CAD build for the part. Positions are in the model's coordinates, mm. A direction names the side the tool comes from. Round coordinates to 2 decimals unless told otherwise and drop trailing zeros. Write each loop counter-clockwise with the first axis right and the second up, starting at its lowest first coordinate (ties: lowest second). Pieces come first, ordered by that corner, then holes. Notation, with made-up numbers: (40, 20.25) - (58, 20.25) arc R11 ccw to (58, 29.25) - close; hole circle Ø5 at (39, 6). An arc over 180 degrees is marked (long way). Use one line per item in the form item = value. Start each with the question number.
Item 1: Band-saw the part on C-C, the plane x = 19.05. List the corners of the cut face in (y, z), and give its area (3 significant figures).
Item 2: Band-saw the part on B-B, the plane z = 0. List the corners of the cut face in (x, y), and give its area (3 significant figures).
Item 3: Pull direction X, two halves, no side cores. Call faces 1 (the cylindrical face through (-23.046, 6.465, 0.176)), 2 (the flat face through (0, 9, 15)), 3 (the flat face through (-24, 2, 0)): +X half, -X half, draft (parallel to the pull), parting line (faces both ways), or undercut.
Item 4: Drill centre lines: L1, parallel to X at y = 2.25, z = 0; L2, parallel to Z at x = 19.05, y = 5.25; L3, parallel to Z at x = -12.5, y = 2.4. Where is each one in solid material? Low to high.
Item 5: Pin check, flat tips, straight feed: pin 1 (4.5 mm diameter, centred on x = 12.5, z = 4, fed in from -Y); pin 2 (2.5 mm diameter, centred on y = 5.5, z = -16, fed in from -X); pin 3 (2.5 mm diameter, centred on y = 7.5, z = 15, fed in from +X). Stop position of each tip, or through.
Item 6: Tool access for faces 4 (the cylindrical face through (10.502, 2.246, 5.088)), 5 (the flat face through (-2.5, 6, 15)), 6 (the flat face through (0, 6, -12.5)), 7 (the flat face through (2.5, 6, 15)), 8 (the cylindrical face through (15.876, 6.465, -2.434)): list every direction of +Z, -Z, +X, -X, +Y, -Y with a clear straight run to the whole face (end or side of a thin tool).
Item 7: Band-saw the part on D-D, the plane z = -5. List the corners of the cut face in (x, y).
Item 8: Band-saw the part on A-A, the plane y = 3.25. List the corners of the cut face in (x, z), and give its area (3 significant figures).
Autodesk Inventor part; units mm, degrees
ref_plane "YZ Plane" through (0, 0, 0) normal (1, 0, 0) x (0, 1, 0)
ref_plane "XZ Plane" through (0, 0, 0) normal (0, 1, 0) x (-1, 0, 0)
ref_plane "XY Plane" through (0, 0, 0) normal (0, 0, 1) x (1, 0, 0)
sketch "Sketch1" plane through (0, 0, 0) normal (0, 1, 0) x (-1, 0, 0)
  line L0 (-24, 17.5) -> (24, 17.5)
  line L1 (24, 17.5) -> (24, -17.5)
  line L2 (24, -17.5) -> (-24, -17.5)
  line L3 (-24, -17.5) -> (-24, 17.5)
  line L4 (-24, 17.5) -> (24, -17.5) construction
  line L5 (24, 17.5) -> (-24, -17.5) construction
  point P0 (0, 0)
  dimension "d0" = 48
  dimension "d1" = 35
extrude "Extrusion1" add sketch "Sketch1" along normal blind 4
sketch "Sketch2" plane through (0, 4, 0) normal (0, 1, 0) x (1, 0, 0)
  line L0 (0, 0) -> (-5.2635, 0) construction
  line L1 (-5.2635, 0) -> (-5.2635, 9.5172) construction
  line L2 (-5.2635, 9.5172) -> (0, 9.5172) construction
  line L3 (0, 9.5172) -> (0, 0) construction
  circle A0 centre (-19.05, 0) radius 1
  circle A1 centre (19.05, 0) radius 1
  circle A2 centre (-19.05, 0) radius 4
  circle A3 centre (19.05, 0) radius 4
  line L4 (-24, -17.5) -> (24, -17.5)
  line L5 (0, -17.5) -> (-2.5, -17.5)
  line L6 (-2.5, -17.5) -> (-2.5, -12.5)
  line L7 (-2.5, -12.5) -> (0, -12.5)
  line L8 (0, -12.5) -> (0, -17.5)
  line L9 (2.5, -17.5) -> (2.5, -12.5)
  line L10 (2.5, -12.5) -> (0, -12.5)
  line L11 (-2.5, 17.5) -> (-2.5, 12.5)
  line L12 (-2.5, 12.5) -> (0, 12.5)
  line L13 (2.5, 17.5) -> (2.5, 12.5)
  line L14 (2.5, 12.5) -> (0, 12.5)
  line L15 (24, 17.5) -> (-24, 17.5)
  dimension "d4" = 2
  dimension "d5" = 19.05
  dimension "d6" = 3
  dimension "d7" = 3
  dimension "d8" = 2.5
  dimension "d9" = 5
extrude "Extrusion2" add sketch "Sketch2" along normal blind 5
chamfer "Chamfer1" distance 15 angle 45 4 edges at (24, 2, -17.5) (24, 2, 17.5) (-24, 2, 17.5) (-24, 2, -17.5)
sketch "Sketch4" plane through (19.05, 9, 0) normal (0, 1, 0) x (1, 0, 0)
  circle A0 centre (0, 0) radius 1
  circle A1 centre (-38.1, 0) radius 1
  point P0 (-19.05, 0)
extrude "Extrusion3" cut sketch "Sketch4" against normal through all
sketch "Sketch7" plane through (0, 0, 0) normal (0, -1, 0) x (1, 0, 0)
  line L0 (14.5, -3) -> (10.5, -3)
  line L1 (10.5, -3) -> (10.5, -7)
  line L2 (10.5, -7) -> (14.5, -7)
  line L3 (14.5, -7) -> (14.5, -3)
  line L4 (0, -6.5734) -> (0, 0) construction
  line L5 (0, 0) -> (6.1677, 0) construction
  line L6 (-14.5, -3) -> (-10.5, -3)
  line L7 (-10.5, -3) -> (-10.5, -7)
  line L8 (-10.5, -7) -> (-14.5, -7)
  line L9 (-14.5, -7) -> (-14.5, -3)
  line L10 (14.5, 3) -> (10.5, 3)
  line L11 (10.5, 3) -> (10.5, 7)
  line L12 (10.5, 7) -> (14.5, 7)
  line L13 (14.5, 7) -> (14.5, 3)
  line L14 (-10.5, 7) -> (-14.5, 7)
  line L15 (-10.5, 3) -> (-10.5, 7)
  line L16 (-14.5, 3) -> (-10.5, 3)
  line L17 (-14.5, 7) -> (-14.5, 3)
  circle A0 centre (12.5, -5) radius 2
  circle A1 centre (-12.5, -5) radius 2
  circle A2 centre (12.5, 5) radius 2
  circle A3 centre (-12.5, 5) radius 2
  point P0 (12.5, -7)
  point P1 (10.5, -5)
  point P2 (12.5, 7)
  point P3 (10.5, 5)
  point P4 (12.5, -3)
  dimension "d30" = 12.5
  dimension "d31" = 4
  dimension "d32" = 4
  dimension "d33" = 5
extrude "Extrusion6" cut sketch "Sketch7" against normal blind 2.5 contours A0 | A1 | A2 | A3
chamfer "Chamfer3" distance 1.5 distance2 2 4 edges at (10.5, 0, 5) (10.5, 0, -5) (-14.5, 0, -5) (-14.5, 0, 5) measured on face at (3, 0, -9.7863)
chamfer "Chamfer4" distance 2 angle 45 2 edges at (-20.05, 9, 0) (18.05, 9, 0)
equation "\"d32\" = d31"
properties part number "Base"
Determined:
q1.outline = (0, -7.45) - (4, -7.45) - (4, -4) - (9, -4) - (9, -3) - (7, -1) - (0, -1) - close; (0, 1) - (7, 1) - (9, 3) - (9, 4) - (4, 4) - (4, 7.45) - (0, 7.45) - close
q1.area = 77.6 mm²
q2.outline = (-24, 0) - (-20.05, 0) - (-20.05, 7) - (-22.05, 9) - (-23.05, 9) - (-23.05, 4) - (-24, 4) - close; (-18.05, 0) - (18.05, 0) - (18.05, 7) - (16.05, 9) - (15.05, 9) - (15.05, 4) - (-15.05, 4) - (-15.05, 9) - (-16.05, 9) - (-18.05, 7) - close; (20.05, 0) - (24, 0) - (24, 4) - (23.05, 4) - (23.05, 9) - (22.05, 9) - (20.05, 7) - close
q2.area = 228 mm²
q3.face_1 = undercut
q3.face_2 = draft
q3.face_3 = -X half
q4.L1 = -24 to -20.05, -18.05 to 18.05, 20.05 to 24
q4.L2 = -4 to -1, 1 to 4
q4.L3 = -14 to -7, -3 to 3, 7 to 14
q5.pin_1 = 0.33
q5.pin_2 = -2.5
q5.pin_3 = 2.5
q6.face_4 = -Y
q6.face_5 = +Z, -Z, -X, +Y
q6.face_6 = +X, -X, +Y
q6.face_7 = +Z, -Z, +X, +Y
q6.face_8 = +Y
q7.outline = (-21.5, 0) - (-16, 0) - (-14.5, 2) - (-14.5, 2.5) - (-10.5, 2.5) - (-10.5, 2) - (-9, 0) - (9, 0) - (10.5, 2) - (10.5, 2.5) - (14.5, 2.5) - (14.5, 2) - (16, 0) - (21.5, 0) - (21.5, 4) - (-21.5, 4) - close
q8.outline = (-24, -2.5) - (-9, -17.5) - (9, -17.5) - (24, -2.5) - (24, 2.5) - (9, 17.5) - (-9, 17.5) - (-24, 2.5) - close; hole circle Ø2 at (-19.05, 0); hole circle Ø2 at (19.05, 0)
q8.area = 1,220 mm²
